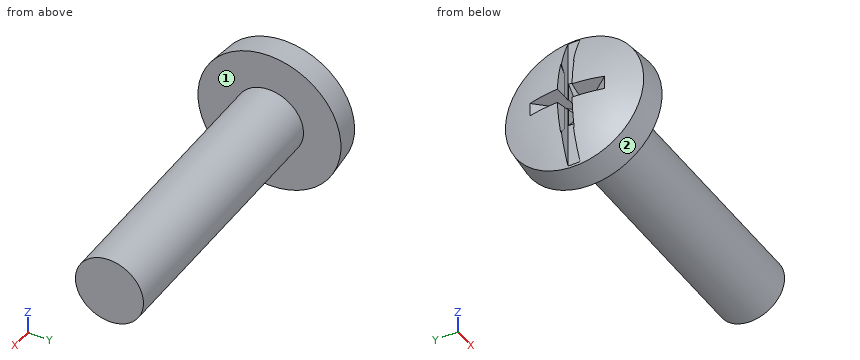
```python
from build123d import *

# Parameters (mm, degrees)
SKETCH2_W         = 20.0152
SKETCH2_H         = 1.7018
SLOT_DEPTH        = 2.2606
CIRPATTERN1_COUNT = 2
CIRPATTERN1_ANGLE = 90


with BuildPart() as part:
    # BodySke → Base-Revolve (revolve)
    with BuildSketch(Plane.XY, mode=Mode.PRIVATE) as base_revolve_sk:
        with BuildLine():
            Line((6.1976, 4.7625), (6.1976, 10.0076))
            Line((6.1976, 10.0076), (2.3876, 9.674268192))
            ThreePointArc((2.3876, 9.674268192), (0.605722555, 4.982271039), (0, 0))
            Line((0, 0), (44.2976, 0))
            Line((44.2976, 0), (44.2976, 4.7625))
            Line((44.2976, 4.7625), (6.1976, 4.7625))
        make_face()
    revolve(base_revolve_sk.sketch.rotate(Axis((-25.4, 0, 0), (1, 0, 0)), 90), axis=Axis((-25.4, 0, 0), (1, 0, 0)))

    # Sketch2 → Slot (cut)
    with BuildSketch(Plane(origin=(0, 0, 0), x_dir=(0, 0, -1), z_dir=(1, 0, 0))):
        Rectangle(SKETCH2_W, SKETCH2_H)
    extrude(amount=SLOT_DEPTH, mode=Mode.SUBTRACT)

    # Sketch3 → Cross section 0
    with BuildSketch(Plane(origin=(0, 0, 0), x_dir=(0, 0, -1), z_dir=(1, 0, 0))):
        with BuildLine():
            Line((-1.0287, 6.096), (1.0287, 6.096))
            Line((1.0287, 6.096), (1.0287, -6.096))
            Line((1.0287, -6.096), (-1.0287, -6.096))
            Line((-1.0287, -6.096), (-1.0287, 6.096))
        make_face()
    # Sketch4 → Cross section 1
    with BuildSketch(Plane(origin=(4.3434, 0, 0), x_dir=(0, 0, -1), z_dir=(1, 0, 0))):
        with BuildLine():
            Line((-0.51435, 0.51435), (0.51435, 0.51435))
            Line((0.51435, 0.51435), (0.51435, -0.51435))
            Line((0.51435, -0.51435), (-0.51435, -0.51435))
            Line((-0.51435, -0.51435), (-0.51435, 0.51435))
        make_face()
    cross = loft(mode=Mode.SUBTRACT)

    # CirPattern1: Cross ×2 about axis
    cirpattern1_axis = Axis((0, 0, 0), (1, 0, 0))
    for i in range(1, CIRPATTERN1_COUNT):
        add(cross.rotate(cirpattern1_axis, i * CIRPATTERN1_ANGLE / (CIRPATTERN1_COUNT - 1)), mode=Mode.SUBTRACT)


solid = part.part
```
Source: CAD feature listing. Evaluate the final solid. Frame: model axes, mm. Face numbers are marked on the shaded views. A direction names the side the tool comes from. Round coordinates to 2 decimals unless told otherwise and drop trailing zeros. Loops run counter-clockwise (first coordinate to the right, second up) from the corner with the lowest first, then second, coordinate; pieces in that order, holes last.
(1) Section query A-A (x = 37.5). Output: boundary loops of the cut face in (y, z) (1 decimal), and give its area (3 significant figures).
From the geometry:
outline: circle Ø9.5 at (0, 0)
area: 71.3 mm2
(2) Access query for the marked faces 1 and 2. Directions: +Z, -Z, +X, -X, +Y, -Y. A direction counts if a zero-diameter tool reaches every point of the face in a straight line with its end or side. Return the directions, or none.
From the geometry:
face 1: +X
face 2: -X
(3) Material intervals for probe 1 along X at (y, z) = (-3.5, -4); probe 2 along Z at (x, y) = (21.5, 0.25); probe 3 along Z at (x, y) = (23, 4.25), sorted ascending.
From the geometry:
probe 1: x = 0.69 to 6.2
probe 2: z = -4.76 to 4.76
probe 3: z = -2.15 to 2.15
(4) Contact query for flat-ended pins moving along their axis: pin 1 Ø0.5 at (y, z) = (0, -5) entering from -X; pin 2 Ø1.9 at (y, z) = (-0.5, 5.5) entering from -X; pin 3 Ø0.5 at (y, z) = (0, 0) entering from -X. Output: stop coordinate, or through.
From the geometry:
pin 1: stops at x = 2.26
pin 2: stops at x = 0.55
pin 3: stops at x = 4.34
